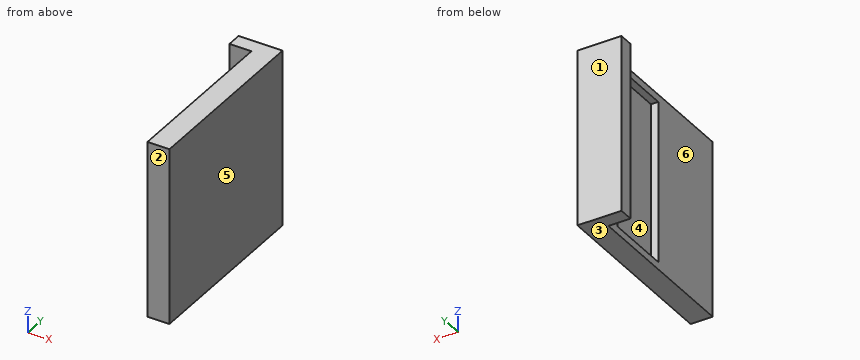
```python
from build123d import *

# Parameters (mm, degrees)
SKETCH1_W           = 3
SKETCH1_H           = 24
BOSS_EXTRUDE1_DEPTH = 23
SKETCH2_W           = 6
SKETCH2_H           = 24
BOSS_EXTRUDE2_DEPTH = 2
SKETCH3_W           = 22
SKETCH3_H           = 9
CUT_EXTRUDE1_DEPTH  = 1


with BuildPart() as part:
    # Sketch1 → Boss-Extrude1 (new body)
    with BuildSketch(Plane(origin=(0, 0, 0), x_dir=(1, 0, 0), z_dir=(0, 1, 0))):
        with Locations((1.5, 12)):
            Rectangle(SKETCH1_W, SKETCH1_H)
    extrude(amount=BOSS_EXTRUDE1_DEPTH)

    # Sketch2 → Boss-Extrude2 (add)
    with BuildSketch(Plane(origin=(0, 23, 0), x_dir=(1, 0, 0), z_dir=(0, 1, 0))):
        with Locations((0, 12)):
            Rectangle(SKETCH2_W, SKETCH2_H)
    extrude(amount=BOSS_EXTRUDE2_DEPTH)

    # Sketch3 → Cut-Extrude1 (cut)
    with BuildSketch(Plane.ZY):
        with Locations((-12, 16.5)):
            Rectangle(SKETCH3_W, SKETCH3_H)
    extrude(amount=-CUT_EXTRUDE1_DEPTH, mode=Mode.SUBTRACT)


solid = part.part
```
The listing builds one solid part. Answer for the finished solid, in the listing's coordinates (mm). Face numbers are marked on the shaded views. A direction names the side the tool comes from. Give positions to 0.01 mm unless a question says otherwise; leave off trailing zeros. Loops run counter-clockwise (first coordinate to the right, second up) from the corner with the lowest first, then second, coordinate; pieces in that order, holes last. Notation, with made-up numbers: M 87,27 L 113,27 A18 cw 113,60 Z; hole C 63,23.25 d2. An arc over 180 degrees is marked long. One line per item, written item: value.
1. Each of these flat-tipped pins is pushed along its axis until it touches: P1, Ø2, axis at y = 13.5, z = -19.5, coming from the -X side; P2, Ø5, axis at y = 8, z = -5.5, coming from the -X side; P3, Ø1.5, axis at x = -2, z = -8, coming from the -Y side. Where does it stop, or does it pass through?
Found:
P1: x = 1
P2: x = 0
P3: y = 23
2. For the marked faces 5 and 6, determine the directions among +Z, -Z, +X, -X, +Y, -Y from which every point of the face is accessible in a straight line to the end or side of a thin tool.
Found:
face 5: +Z, -Z, +X, +Y, -Y
face 6: +Z, -Z, -X, -Y
3. For a pull along Y with two mould halves and no side action, classify the marked faces 1, 2, 3 and 4 as pulls with the +Y half, pulls with the -Y half, needs draft (parallel to the pull), parting line crosses it, or undercut.
Found:
face 1: pulls with the +Y half
face 2: pulls with the -Y half
face 3: needs draft
face 4: undercut
4. Section D-D on y = 3.25 is taken. Determine the outline of the cut face in (x, z), plus the area to 3 significant figures.
Found:
outline: M 0,-24 L 3,-24 L 3,0 L 0,0 Z
area: 72.0 mm^2
5. Section C-C on x = -1.8 is taken. Determine the outline of the cut face in (y, z), plus the area to 3 significant figures.
Found:
outline: M 23,-24 L 25,-24 L 25,0 L 23,0 Z
area: 48.0 mm^2
6. Find the intervals of material crossed by probe 1 along Y at (x, z) = (0.4, -5.5); probe 2 along X at (y, z) = (22.25, -11.5); probe 3 along X at (y, z) = (20.5, -10.5), in increasing order.
Found:
probe 1: 0 to 12, 21 to 25
probe 2: 0 to 3
probe 3: 1 to 3
7. Section A-A on y = 13.5 is taken. Determine the outline of the cut face in (x, z).
Found:
outline: M 0,-24 L 3,-24 L 3,0 L 0,0 L 0,-1 L 1,-1 L 1,-23 L 0,-23 Z
8. Section B-B on z = -17.25 is taken. Determine the outline of the cut face in (x, y), plus the area to 3 significant figures.
Found:
outline: M -3,23 L 0,23 L 0,21 L 1,21 L 1,12 L 0,12 L 0,0 L 3,0 L 3,25 L -3,25 Z
area: 72.0 mm^2
